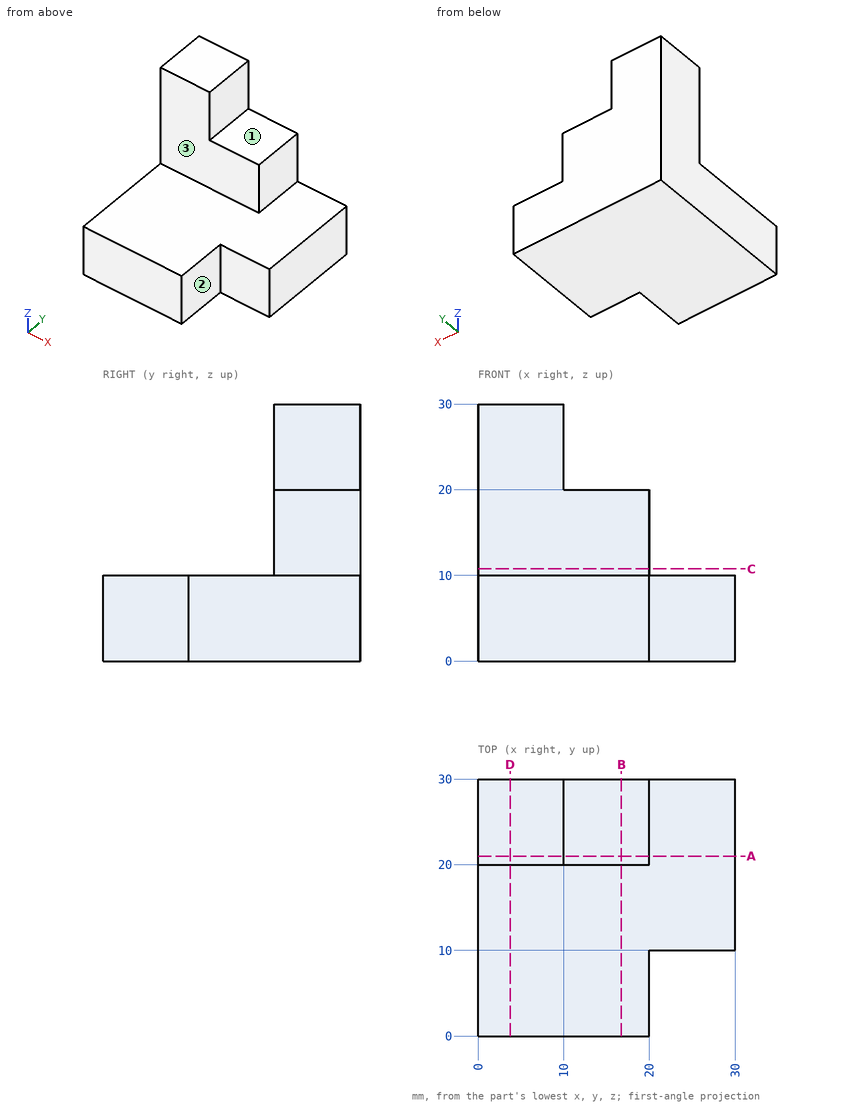
Answer from the drawing. Dimensions are ordinates in mm from the lowest x, y and z of the part. A direction names the side the tool comes from. Coordinates: 2 decimals unless noted, no trailing zeros. Write each loop counter-clockwise with the first axis right and the second up, starting at its lowest first coordinate (ties: lowest second). Pieces come first, ordered by that corner, then holes. Notation, with made-up numbers: M 34,74.25 L 82,74.25 A35 ccw 82,107.25 Z; hole C -14.75,-23 d1. An arc over 180 degrees is marked long. Put each result on its own line as item: value. Start each with the question number.
1. A cutting plane is placed at A-A on y = 21. Write down the section's boundary in (x, z), then the cut area to 3 significant figures.
2. Consider line 1 (X direction, y = 25.5, z = 17); line 2 (Z direction, x = 5.25, y = 6.75); line 3 (Y direction, x = 3.5, z = 10.75). Determine where each line is inside the solid, lowest interval first. Write a range as from..to.
3. A cutting plane is placed at B-B on x = 16.75. Write down the section's boundary in (y, z).
4. Which of the six approach directions +Z, -Z, +X, -X, +Y, -Y give full straight-line access (tool end or side, diameter ignored) to the marked faces 1, 2 and 3?
5. A cutting plane is placed at C-C on z = 10.75. Write down the section's boundary in (x, y), then the cut area to 3 significant figures.
6. A cutting plane is placed at D-D on x = 3.75. Write down the section's boundary in (y, z), then the cut area to 3 significant figures.
7. Flat-ended cylindrical pins translate along their axes: P1, Ø5, axis at x = 26, z = 13, coming from the +Y side; P2, Ø5, axis at x = 14.5, y = 12.5, coming from the +Z side; P3, Ø3, axis at y = 23.5, z = 14, coming from the +X side; P4, Ø8, axis at y = 23.5, z = 24.5, coming from the +X side. Find the tip coordinate at first contact, or state that the pin passes through.
Resolved:
1. outline: M 0,0 L 30,0 L 30,10 L 20,10 L 20,20 L 10,20 L 10,30 L 0,30 Z
1. area: 600 mm2
2. line 1: x = 0..20
2. line 2: z = 0..10
2. line 3: y = 20..30
3. outline: M 0,0 L 30,0 L 30,20 L 20,20 L 20,10 L 0,10 Z
4. face 1: +Z, +X, +Y, -Y
4. face 2: +Z, -Z, +X, -Y
4. face 3: +Z, +X, -X, -Y
5. outline: M 0,20 L 20,20 L 20,30 L 0,30 Z
5. area: 200 mm2
6. outline: M 0,0 L 30,0 L 30,30 L 20,30 L 20,10 L 0,10 Z
6. area: 500 mm2
7. P1: passes through
7. P2: stops at z = 10
7. P3: stops at x = 20
7. P4: stops at x = 10
